```python
from build123d import *

# Parameters (mm, degrees)
F1_DEPTH = 25.4
F2_R     = 12.041499
F3_DEPTH = 25.4
F4_R     = 4.250417
F5_DEPTH = 25.401


with BuildPart() as f1:
    # F0 (on Top) → F1 (new body)
    with BuildSketch(Plane.XY):
        with BuildLine():
            ThreePointArc((-15.021411, -7.063877), (-16.521823, 1.603285), (-13.382968, 9.82025))
            Line((-13.382968, 9.82025), (-13.382968, 15.685415))
            ThreePointArc((-13.382968, 15.685415), (-16.512447, 22.126296), (-22.880558, 18.851278))
            ThreePointArc((-22.880558, 18.851278), (-28.833329, 17.93548), (-28.931248, 11.913473))
            Line((-28.931248, 11.913473), (-45.90502, 15.685415))
            Line((-45.90502, 15.685415), (-48.207462, 5.324407))
            Line((-48.207462, 5.324407), (-36.421049, 5.324407))
            Line((-36.421049, 5.324407), (-36.421049, 0))
            Line((-36.421049, 0), (-49.811375, -3.183969))
            Line((-49.811375, -3.183969), (-48.207462, -9.929298))
            Line((-48.207462, -9.929298), (-36.103659, -7.05124))
            Line((-36.103659, -7.05124), (-36.103659, -12.34197))
            Line((-36.103659, -12.34197), (-44.427202, -17.650355))
            Line((-44.427202, -17.650355), (-40.724512, -23.456169))
            Line((-40.724512, -23.456169), (-15.021411, -7.063877))
        make_face()
        with BuildLine():
            ThreePointArc((13.382968, -9.82025), (15.774835, -5.166792), (16.599433, 0))
            ThreePointArc((16.599433, 0), (16.200124, 3.618995), (15.021411, 7.063877))
            ThreePointArc((15.021411, 7.063877), (12.816387, 10.549), (9.82025, 13.382968))
            ThreePointArc((9.82025, 13.382968), (1.603285, 16.521823), (-7.063877, 15.021411))
            ThreePointArc((-7.063877, 15.021411), (-10.549, 12.816387), (-13.382968, 9.82025))
            ThreePointArc((-13.382968, 9.82025), (-16.521823, 1.603285), (-15.021411, -7.063877))
            ThreePointArc((-15.021411, -7.063877), (-12.816387, -10.549), (-9.82025, -13.382968))
            ThreePointArc((-9.82025, -13.382968), (-1.603285, -16.521823), (7.063877, -15.021411))
            ThreePointArc((7.063877, -15.021411), (10.549, -12.816387), (13.382968, -9.82025))
        make_face()
        with BuildLine():
            ThreePointArc((15.021411, 7.063877), (16.200124, 3.618995), (16.599433, 0))
            ThreePointArc((16.599433, 0), (15.774835, -5.166792), (13.382968, -9.82025))
            Line((13.382968, -9.82025), (13.382968, -15.685415))
            ThreePointArc((13.382968, -15.685415), (16.512447, -22.126296), (22.880558, -18.851278))
            ThreePointArc((22.880558, -18.851278), (28.833329, -17.93548), (28.931248, -11.913473))
            Line((28.931248, -11.913473), (45.90502, -15.685415))
            Line((45.90502, -15.685415), (48.207462, -5.324407))
            Line((48.207462, -5.324407), (36.421049, -5.324407))
            Line((36.421049, -5.324407), (36.421049, 0))
            Line((36.421049, 0), (49.811375, 3.183969))
            Line((49.811375, 3.183969), (48.207462, 9.929298))
            Line((48.207462, 9.929298), (36.103659, 7.05124))
            Line((36.103659, 7.05124), (36.103659, 12.34197))
            Line((36.103659, 12.34197), (44.427202, 17.650355))
            Line((44.427202, 17.650355), (40.724512, 23.456169))
            Line((40.724512, 23.456169), (15.021411, 7.063877))
        make_face()
        with BuildLine():
            Line((23.456169, -40.724512), (7.063877, -15.021411))
            ThreePointArc((7.063877, -15.021411), (-1.603285, -16.521823), (-9.82025, -13.382968))
            Line((-9.82025, -13.382968), (-15.685415, -13.382968))
            ThreePointArc((-15.685415, -13.382968), (-22.126296, -16.512447), (-18.851278, -22.880558))
            ThreePointArc((-18.851278, -22.880558), (-17.93548, -28.833329), (-11.913473, -28.931248))
            Line((-11.913473, -28.931248), (-15.685415, -45.90502))
            Line((-15.685415, -45.90502), (-5.324407, -48.207462))
            Line((-5.324407, -48.207462), (-5.324407, -36.421049))
            Line((-5.324407, -36.421049), (0, -36.421049))
            Line((0, -36.421049), (3.183969, -49.811375))
            Line((3.183969, -49.811375), (9.929298, -48.207462))
            Line((9.929298, -48.207462), (7.05124, -36.103659))
            Line((7.05124, -36.103659), (12.34197, -36.103659))
            Line((12.34197, -36.103659), (17.650355, -44.427202))
            Line((17.650355, -44.427202), (23.456169, -40.724512))
        make_face()
        with BuildLine():
            ThreePointArc((-7.063877, 15.021411), (1.603285, 16.521823), (9.82025, 13.382968))
            Line((9.82025, 13.382968), (15.685415, 13.382968))
            ThreePointArc((15.685415, 13.382968), (22.126296, 16.512447), (18.851278, 22.880558))
            ThreePointArc((18.851278, 22.880558), (17.93548, 28.833329), (11.913473, 28.931248))
            Line((11.913473, 28.931248), (15.685415, 45.90502))
            Line((15.685415, 45.90502), (5.324407, 48.207462))
            Line((5.324407, 48.207462), (5.324407, 36.421049))
            Line((5.324407, 36.421049), (0, 36.421049))
            Line((0, 36.421049), (-3.183969, 49.811375))
            Line((-3.183969, 49.811375), (-9.929298, 48.207462))
            Line((-9.929298, 48.207462), (-7.05124, 36.103659))
            Line((-7.05124, 36.103659), (-12.34197, 36.103659))
            Line((-12.34197, 36.103659), (-17.650355, 44.427202))
            Line((-17.650355, 44.427202), (-23.456169, 40.724512))
            Line((-23.456169, 40.724512), (-7.063877, 15.021411))
        make_face()
    extrude(amount=F1_DEPTH)

    # F2 (on face) → F3 (cut)
    with BuildSketch(Plane.XY.offset(25.4)):
        Circle(F2_R)
    extrude(amount=-F3_DEPTH, mode=Mode.SUBTRACT)

    # F4 (on face) → F5 (cut, through all)
    with BuildSketch(Plane.XY.offset(25.4)):
        with Locations((11.656133, 20.290306)):
            Circle(F4_R)
    extrude(amount=-F5_DEPTH, mode=Mode.SUBTRACT)


solid = f1.part
```
Model file for the job. Use its own axes, mm. A direction names the side the tool comes from. Give positions to 0.01 mm unless a question says otherwise; leave off trailing zeros. Write each loop counter-clockwise with the first axis right and the second up, starting at its lowest first coordinate (ties: lowest second). Pieces come first, ordered by that corner, then holes. Notation, with made-up numbers: M -8.75,22.25 L 39.25,22.25 A28 cw 39.25,53.25 Z; hole C 42.5,52 d1. An arc over 180 degrees is marked long. Use a Markdown table: item, result.
1) Cut at C-C (x = -43). List the corners of the cut face in (y, z).
Responses:
| item | result |
|---|---|
| outline | M -19.89,0 L -16.74,0 L -16.74,25.4 L -19.89,25.4 Z; M -8.69,0 L -1.56,0 L -1.56,25.4 L -8.69,25.4 Z; M 5.32,0 L 15.04,0 L 15.04,25.4 L 5.32,25.4 Z |
2) Cut at A-A (y = -8.5). List the corners of the cut face in (x, z), and give its area (3 significant figures).
Responses:
| item | result |
|---|---|
| outline | M -48.55,0 L -42.2,0 L -42.2,25.4 L -48.55,25.4 Z; M -36.1,0 L -17.27,0 L -17.27,25.4 L -36.1,25.4 Z; M -14.26,0 L -8.53,0 L -8.53,25.4 L -14.26,25.4 Z; M 8.53,0 L 47.5,0 L 47.5,25.4 L 8.53,25.4 Z |
| area | 1,780 mm2 |
3) Cut at D-D (z = 12). Give the number of separate pieces and of enclosed holes in the cut face, and give its area (3 significant figures).
Responses:
| item | result |
|---|---|
| separate pieces | 1 |
| enclosed holes | 2 |
| area | 4,060 mm2 |
4) Pin check, flat tips, straight feed: pin 1 (2.5 mm diameter, centred on x = -2.5, z = 16.5, fed in from -Y); pin 2 (4.5 mm diameter, centred on y = -3.5, z = 19, fed in from +X); pin 3 (2.5 mm diameter, centred on x = -11, z = 9, fed in from +Y). Stop position of each tip, or through.
Responses:
| item | result |
|---|---|
| pin 1 | stops at y = -36.42 |
| pin 2 | stops at x = 48.21 |
| pin 3 | stops at y = 48.25 |
5) Tool access for faces 1 (the flat face through (-49.02, -6.51, 12.52)), 2 (the flat face through (36.104, 10, 13)), 3 (the flat face through (40.21, 14.96, 12.52)): list every direction of +Z, -Z, +X, -X, +Y, -Y with a clear straight run to the whole face (end or side of a thin tool).
Responses:
| item | result |
|---|---|
| face 1 | +Z, -Z, -X, -Y |
| face 2 | +Z, -Z |
| face 3 | +Z, -Z, +X |
6) Cut at B-B (x = 39). List the corners of the cut face in (y, z), and give its area (3 significant figures).
Responses:
| item | result |
|---|---|
| outline | M -14.15,0 L -5.32,0 L -5.32,25.4 L -14.15,25.4 Z; M 0.61,0 L 7.74,0 L 7.74,25.4 L 0.61,25.4 Z; M 14.19,0 L 22.36,0 L 22.36,25.4 L 14.19,25.4 Z |
| area | 613 mm2 |
7) Pull direction Y, two halves, no side cores. Call faces 4 (the cylindrical face through (-9.556, -7.327, 12.878)), 5 (the flat face through (-11, 8, 25.4)), 6 (the flat face through (3, 36.421, 13)): +Y half, -Y half, draft (parallel to the pull), parting line (faces both ways), or undercut.
Responses:
| item | result |
|---|---|
| face 4 | undercut |
| face 5 | draft |
| face 6 | +Y half |
8) Drill centre lines: line 1 (Y direction, x = 21, z = 10); line 2 (X direction, y = 18.5, z = 3); line 3 (Y direction, x = -44, z = 17.25). Where is each one in solid material? Low to high. Write a range as from..to.
Responses:
| item | result |
|---|---|
| line 1 | y = -42.29..-36.87, -21.45..10.88, 14.64..21.55 |
| line 2 | x = -28.25..-13.22, -9.28..7.8, 15.51..22.37, 32.95..43.89 |
| line 3 | y = -18.32..-17.38, -8.93..-1.8, 5.32..15.26 |
